Can you work these out from the model? Positions are in its coordinate system, mm. Coordinates: 2 decimals unless noted, no trailing zeros. Order: outer loops, then holes, each group sorted by start corner. A loop starts at its lowest first (then second) coordinate and runs counter-clockwise, first axis right, second up.
```python
from build123d import *

# Parameters (mm, degrees)
F1_DEPTH = 5
F3_D     = 22
F5_D     = 22
F7_D     = 22


with BuildPart() as f1:
    # F0 (on Top) → F1 (new body)
    with BuildSketch(Plane.XY):
        with BuildLine():
            ThreePointArc((14.439225008, -4.5701776484), (13.7453052389, 0), (14.439225008, 4.5701776484))
            ThreePointArc((14.4392250081, 4.5701776484), (0.116311071, 15.1447751487), (-14.3673285073, 4.7914104535))
            ThreePointArc((-14.3673285073, 4.7914104535), (-13.7951814402, 2.4260059517), (-13.602864396, 0))
            ThreePointArc((-13.602864396, 0), (-13.7951814402, -2.4260059517), (-14.3673285073, -4.7914104535))
            ThreePointArc((-14.3673285073, -4.7914104535), (0.116311071, -15.1447751487), (14.4392250081, -4.5701776484))
        make_face()
        with BuildLine():
            ThreePointArc((-14.3673285073, -4.7914104535), (-15.1452217736, 0), (-14.3673285073, 4.7914104535))
            ThreePointArc((-14.3673285073, 4.7914104535), (-19.7467605123, 12.306770976), (-28.4601684953, 15.3882403981))
            Line((-28.4601684953, 15.3882403981), (-29.545495717, 15.3880823672))
            ThreePointArc((-29.545495717, 15.3880823672), (-44.3915356245, -0.4569880798), (-28.6315344711, -15.3933036246))
            ThreePointArc((-28.6315344711, -15.3933036246), (-19.8154166919, -12.3580970844), (-14.3673285073, -4.7914104535))
        make_face()
        with BuildLine():
            ThreePointArc((29.1410469099, -15.3966274615), (20.0122054796, -12.3977505372), (14.439225008, -4.5701776484))
            ThreePointArc((14.4392250081, -4.5701776484), (0.116311071, -15.1447751487), (-14.3673285073, -4.7914104535))
            ThreePointArc((-14.3673285073, -4.7914104535), (-19.8154166919, -12.3580970844), (-28.6315344711, -15.3933036246))
            Line((-28.6315344711, -15.3933036246), (29.1410469099, -15.3966274615))
        make_face()
        with BuildLine():
            ThreePointArc((-14.3673285073, 4.7914104535), (0.116311071, 15.1447751487), (14.4392250081, 4.5701776484))
            ThreePointArc((14.439225008, 4.5701776484), (20.0116595313, 12.3973484813), (29.1396908737, 15.3966273238))
            Line((29.1396908737, 15.3966273238), (-28.4601684953, 15.3882403981))
            ThreePointArc((-28.4601684953, 15.3882403981), (-19.7467605123, 12.306770976), (-14.3673285073, 4.7914104535))
        make_face()
        with BuildLine():
            ThreePointArc((14.4392250081, 4.5701776484), (14.9676819774, 2.3121935024), (15.1452217736, 0))
            ThreePointArc((15.1452217736, 0), (14.9676819774, -2.3121935024), (14.4392250081, -4.5701776484))
            ThreePointArc((14.439225008, -4.5701776484), (20.0122054796, -12.3977505372), (29.1410469099, -15.3966274615))
            ThreePointArc((29.1410469099, -15.3966274615), (40.0286792416, -10.8873728822), (44.5385602129, 0))
            ThreePointArc((44.5385602129, 0), (40.0281997861, 10.8878522891), (29.1396908737, 15.3966273238))
            ThreePointArc((29.1396908737, 15.3966273238), (20.0116595313, 12.3973484813), (14.439225008, 4.5701776484))
        make_face()
    extrude(amount=F1_DEPTH)

    # F3 (through all)
    with Locations(Plane.XY.offset(5)):
        with Locations((-29.0005914867, 0)):
            Hole(F3_D / 2)

    # F5 (through all)
    with Locations(Plane.XY.offset(5)):
        with Locations((0, 0)):
            Hole(F5_D / 2)

    # F7 (through all)
    with Locations(Plane.XY.offset(5)):
        with Locations((29.1419327259, 0)):
            Hole(F7_D / 2)


solid = f1.part
```
1. Imagine slicing it at A-A on y = 1. Please give me the cut outline in (x, z), then the cut area to 3 significant figures.
Completed:
outline: (-44.37, 0) - (-39.96, 0) - (-39.96, 5) - (-44.37, 5) - close; (-18.05, 0) - (-15.11, 0) - (-15.11, 5) - (-18.05, 5) - close; (-13.64, 0) - (-10.95, 0) - (-10.95, 5) - (-13.64, 5) - close; (10.95, 0) - (13.78, 0) - (13.78, 5) - (10.95, 5) - close; (15.11, 0) - (18.19, 0) - (18.19, 5) - (15.11, 5) - close; (40.1, 0) - (44.51, 0) - (44.51, 5) - (40.1, 5) - close
area: 102 mm2
2. Imagine slicing it at C-C on x = -6.5. Please give me the cut outline in (y, z), then the cut area to 3 significant figures.
Completed:
outline: (-15.39, 0) - (-8.87, 0) - (-8.87, 5) - (-15.39, 5) - close; (8.87, 0) - (15.39, 0) - (15.39, 5) - (8.87, 5) - close
area: 65.2 mm2
3. I'm going to push flat-ended pins straight in: pin 1 (2 mm diameter, centred on x = -14, z = 1, fed in from -Y); pin 2 (6 mm diameter, centred on x = 22.5, y = -6.5, fed in from -Z); pin 3 (1.5 mm diameter, centred on y = 9, z = 2.5, fed in from +X). Where does each tip first touch, or does it pass through?
Completed:
pin 1: stops at y = -15.39
pin 2: stops at z = 0
pin 3: stops at x = 42.14
4. Imagine slicing it at B-B on z = 2.35. Please give me the cut outline in (x, y), then the cut area to 3 significant figures.
Completed:
outline: (-29.55, 15.39) arc R15.4 ccw to (-28.63, -15.39) - (29.14, -15.4) arc R15.4 ccw to (29.14, 15.4) - close; hole circle Ø22 at (-29, 0); hole (-14.37, -4.79) arc R15.4 ccw to (-14.37, 4.79) arc R15.15 ccw to start; hole circle Ø22 at (0, 0); hole (14.44, -4.57) arc R15.15 ccw to (14.44, 4.57) arc R15.4 ccw to start; hole circle Ø22 at (29.14, 0)
area: 1,380 mm2
5. Thinking about a two-plate mould opening in X: for faces 1 (the cylindrical face through (-26.62, -10.74, 2.47)), 2 (the flat face through (-10, 7, 5)), 3 (the cylindrical face through (13.745, -0.065, 2.465)), which applies, pulls with the +X half, pulls with the -X half, needs draft (parallel to the pull), parting line crosses it, or undercut?
Completed:
face 1: undercut
face 2: needs draft
face 3: undercut
6. Please list where these lines run through material, in increasing order: probe 1 along X at (y, z) = (-9.5, 3.1); probe 2 along Y at (x, z) = (29, 1.4); probe 3 along X at (y, z) = (-8, 2.1).
Completed:
probe 1: x = -41.12 to -34.55, -23.46 to -5.55, 5.55 to 23.6, 34.69 to 41.26
probe 2: y = -15.4 to -11, 11 to 15.4
probe 3: x = -42.16 to -36.55, -21.45 to -7.55, 7.55 to 21.59, 36.69 to 42.3
7. Imagine slicing it at D-D on y = -7. Please give me the cut outline in (x, z), then the cut area to 3 significant figures.
Completed:
outline: (-42.72, 0) - (-37.49, 0) - (-37.49, 5) - (-42.72, 5) - close; (-20.52, 0) - (-8.49, 0) - (-8.49, 5) - (-20.52, 5) - close; (8.49, 0) - (20.66, 0) - (20.66, 5) - (8.49, 5) - close; (37.63, 0) - (42.86, 0) - (42.86, 5) - (37.63, 5) - close
area: 173 mm2
